Work out the finished part from the listing and answer in its coordinate system (mm). A direction names the side the tool comes from. Round coordinates to 2 decimals unless told otherwise and drop trailing zeros. Write each loop counter-clockwise with the first axis right and the second up, starting at its lowest first coordinate (ties: lowest second). Pieces come first, ordered by that corner, then holes. Notation, with made-up numbers: (76, 4.25) -> (82, 4.25) arc R18 ccw to (82, 26.25) -> close; hole circle Ø6 at (11.5, -25). An arc over 180 degrees is marked (long way). Answer as a JSON object with one key per item and string values. Group by question number.
from build123d import *

# Parameters (mm, degrees)
SKETCH1_R           = 7.14375
BOSS_EXTRUDE1_DEPTH = 4.445


with BuildPart() as part:
    # Sketch1 → Boss-Extrude1 (new, symmetric)
    with BuildSketch(Plane(origin=(0, 0, 0), x_dir=(1, 0, 0), z_dir=(0, 1, 0))):
        with Locations(Location((0, 0, 0), (0, 0, 270))):
            Circle(SKETCH1_R)
        Polygon((2.786292399, -4.826), (5.572584798, 0), (2.786292399, 4.826), (-2.786292399, 4.826), (-5.572584798, 0), (-2.786292399, -4.826), align=None, mode=Mode.SUBTRACT)
    extrude(amount=BOSS_EXTRUDE1_DEPTH, both=True)


solid = part.part
1) A tool of negligible diameter and unlimited length cuts with its end or side. For faces 4 (the face through (4.2, 0.06, -2.38)), 5 (the face through (0, -4.445, -5)), from which of +Z, -Z, +X, -X, +Y, -Y can it reach the whole face along a straight path? Write none if from no direction.
2) A cutting plane is placed at B-B on y = -1. Determine the outline of the cut face in (x, z).
3) Each of these flat-tipped pins is pushed along its axis until it touches: P1, Ø4.5, axis at x = 1, y = -1, coming from the -Z side; P2, Ø4, axis at y = 2, z = 4.5, coming from the -X side; P3, Ø1, axis at x = 1, y = -2.5, coming from the +Z side; P4, Ø5, axis at y = -1.5, z = -5, coming from the +X side. Where does it stop, or does it pass through?
4) A cutting plane is placed at A-A on x = 0. Determine the outline of the cut face in (y, z) (3 decimals).
5) A cutting plane is placed at C-C on z = 2. Determine the outline of the cut face in (x, y) (3 decimals), plus the area to 3 significant figures.
6) For a pull along Z with two mould halves and no side action, classify faces 1 (the face through (0, 0, -4.826)), 2 (the face through (0.314, 0.062, -7.137)), 3 (the face through (0, 4.445, -5)) as released by +Z, released by -Z, zero draft, split by the parting line, or undercut.
7) Straight lines are drawn through the part: L1, parallel to X at y = -0.75, z = 4.25; L2, parallel to X at y = 4, z = 3.5; L3, parallel to Z at x = 0.5, y = -0.25. For each, find the intervals that lie inside material, in ascending order.
Established:
{
 "1": {"face 4": "+Y, -Y", "face 5": "+Z, -Z, +X, -X, -Y"},
 "2": {"outline": "circle Ø14.29 at (0, 0); hole (-5.57, 0) -> (-2.79, -4.83) -> (2.79, -4.83) -> (5.57, 0) -> (2.79, 4.83) -> (-2.79, 4.83) -> close"},
 "3": {"P1": "stops at z = -7.14", "P2": "stops at x = -6.69", "P3": "stops at z = 7.13", "P4": "stops at x = 6.69"},
 "4": {"outline": "(-4.445, -7.144) -> (4.445, -7.144) -> (4.445, -4.826) -> (-4.445, -4.826) -> close; (-4.445, 4.826) -> (4.445, 4.826) -> (4.445, 7.144) -> (-4.445, 7.144) -> close"},
 "5": {"outline": "(-6.858, -4.445) -> (-4.418, -4.445) -> (-4.418, 4.445) -> (-6.858, 4.445) -> close; (4.418, -4.445) -> (6.858, -4.445) -> (6.858, 4.445) -> (4.418, 4.445) -> close", "area": "43.4 mm²"},
 "6": {"face 1": "undercut", "face 2": "split by the parting line", "face 3": "zero draft"},
 "7": {"L1": "x = -5.74 to -3.12, 3.12 to 5.74", "L2": "x = -6.23 to -3.55, 3.55 to 6.23", "L3": "z = -7.13 to -4.83, 4.83 to 7.13"}
}
